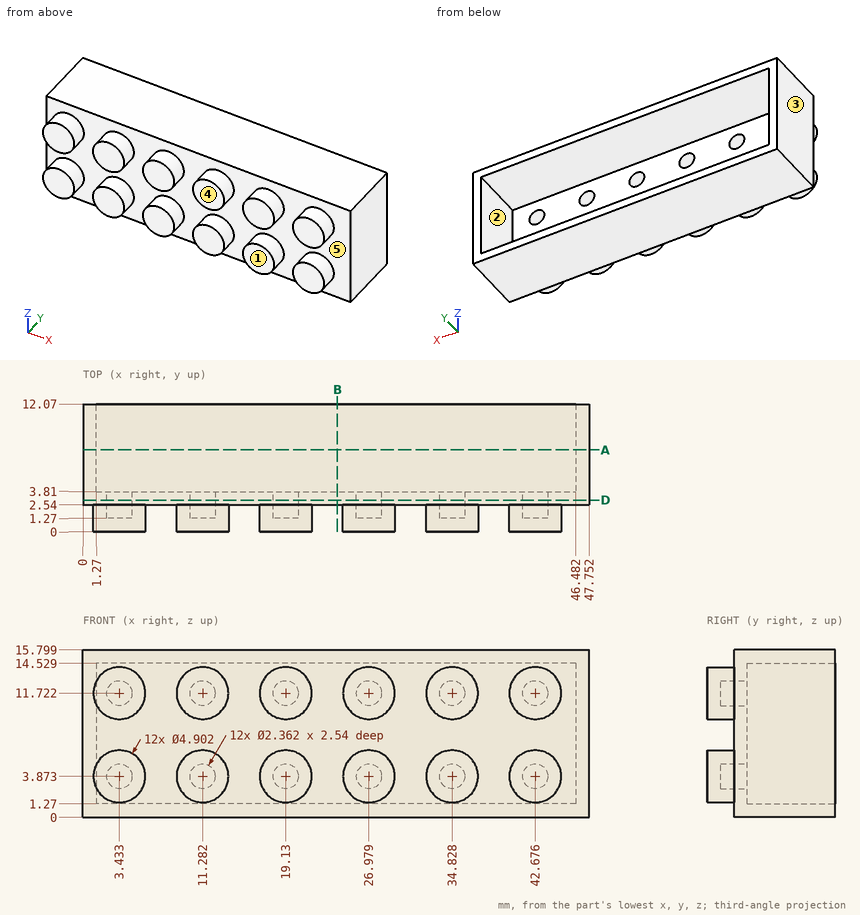
Part print with two shaded views. Sizes in mm from the minimum x, y, z corner. A direction names the side the tool comes from. Round coordinates to 2 decimals unless told otherwise and drop trailing zeros. Loops run counter-clockwise (first coordinate to the right, second up) from the corner with the lowest first, then second, coordinate; pieces in that order, holes last. Notation, with made-up numbers: (31, 84) - (80, 84) arc R22 cw to (80, 120) - close; hole circle Ø10 at (-0.5, 72.5). An arc over 180 degrees is marked (long way). Answer as a JSON object with one key per item and string values.
Item 1: Pin check, flat tips, straight feed: pin 1 (6.5 mm diameter, centred on y = 6.5, z = 10.5, fed in from -X); pin 2 (2.5 mm diameter, centred on x = 11.5, z = 4, fed in from +Y); pin 3 (1.2 mm diameter, centred on x = 42.5, z = 3.5, fed in from +Y); pin 4 (2 mm diameter, centred on x = 39, z = 11.5, fed in from -Y). Stop position of each tip, or through.
Output:
{"pin 1": "x = 0", "pin 2": "y = 3.81", "pin 3": "y = 1.27", "pin 4": "y = 2.54"}
Item 2: Band-saw the part on A-A on y = 7.75. List the corners of the cut face in (x, z), plus the area to 3 significant figures.
Output:
{"outline": "(0, 0) - (47.75, 0) - (47.75, 15.8) - (0, 15.8) - close; hole (1.27, 1.27) - (46.48, 1.27) - (46.48, 14.53) - (1.27, 14.53) - close", "area": "155 mm2"}
Item 3: Band-saw the part on B-B on x = 24. List the corners of the cut face in (y, z).
Output:
{"outline": "(2.54, 0) - (12.07, 0) - (12.07, 1.27) - (3.81, 1.27) - (3.81, 14.53) - (12.07, 14.53) - (12.07, 15.8) - (2.54, 15.8) - close"}
Item 4: Wall check: L1, parallel to Z at x = 5, y = 10; L2, parallel to X at y = 10.75, z = 13.5; L3, parallel to Y at x = 8, z = 14.75. Give the ranges that are in metal, low to high.
Output:
{"L1": "0 to 1.27, 14.53 to 15.8", "L2": "0 to 1.27, 46.48 to 47.75", "L3": "2.54 to 12.07"}
Item 5: Tool access for the marked faces 1 and 2: list every direction of +Z, -Z, +X, -X, +Y, -Y with a clear straight run to the whole face (end or side of a thin tool).
Output:
{"face 1": "+Z, -Z, +X, -X, -Y", "face 2": "+Y"}
Item 6: Band-saw the part on D-D on y = 3. State how many separate pieces and enclosed holes the cut face has, plus the area to 3 significant figures.
Output:
{"separate pieces": "1", "enclosed holes": "12", "area": "702 mm2"}
Item 7: Pull direction X, two halves, no side cores. Call the marked faces 3, 4 and 5: pulls with the +X half, pulls with the -X half, needs draft (parallel to the pull), parting line crosses it, or undercut.
Output:
{"face 3": "pulls with the -X half", "face 4": "needs draft", "face 5": "undercut"}
